from build123d import *

# Parameters (mm, degrees)
F0_W     = 50
F0_H     = 19
F0_H_2   = 13
F0_W_2   = 1.5
F1_DEPTH = 1.5
F2_R     = 0.74999
F4_DEPTH = 1.5
F5_R     = 1.49999
F3_W     = 2
F3_H     = 5
F6_DEPTH = 0.3


# Not quite as in the source:
# - a fillet or chamfer is up to 0.001 mm smaller than in the source, because OpenCascade refuses the exact size


with BuildPart() as f1:
    # F0 (on Top) → F1 (new body)
    with BuildSketch(Plane.XY):
        with Locations((0, -6.5)):
            Rectangle(F0_W, F0_H)
        with Locations((0, 9.5)):
            Rectangle(F0_W, F0_H_2)
        with Locations((-25.75, 9.5)):
            Rectangle(F0_W_2, F0_H_2)
        with Locations((25.75, 9.5)):
            Rectangle(F0_W_2, F0_H_2)
    extrude(amount=F1_DEPTH)

    # F2 (radius 0.75 in the source; OpenCascade refuses exactly that, so slightly less here)
    f2_edges = [f1.edges().sort_by_distance(p)[0] for p in [
        (-26.5, 16, 0.75),
        (-26.5, 3, 0.75),
        (-25, 3, 0.75),
        (-25, -16, 0.75),
        (25, -16, 0.75),
        (25, 3, 0.75),
        (26.5, 3, 0.75),
        (26.5, 16, 0.75),
    ]]
    fillet(f2_edges, radius=F2_R)

    # F3 (on face) → F4 (join)
    with BuildSketch(Plane.XY.offset(1.5)):
        Polygon((-23.5, 2.25), (-25, 2.25), (-25, -15.25), (-23.5, -15.25), (-23.5, -7), (-23.5, -2), align=None)
        Polygon((23.5, -15.25), (25, -15.25), (25, 2.25), (23.5, 2.25), (23.5, -2), (23.5, -7), align=None)
    extrude(amount=F4_DEPTH)

    # F5 (radius 1.5 in the source; OpenCascade refuses exactly that, so slightly less here)
    f5_edges = [f1.edges().sort_by_distance(p)[0] for p in [
        (-23.5, -6.5, 3),
        (23.5, -6.5, 3),
    ]]
    fillet(f5_edges, radius=F5_R)

    # F3 (on face) → F6 (join)
    with BuildSketch(Plane.XY.offset(1.5)):
        with Locations((-22.5, -4.5)):
            Rectangle(F3_W, F3_H)
        with Locations((22.5, -4.5)):
            Rectangle(F3_W, F3_H)
    extrude(amount=F6_DEPTH)


solid = f1.part
Work out the finished part from the listing and answer in its coordinate system (mm). A direction names the side the tool comes from. Give positions to 0.01 mm unless a question says otherwise; leave off trailing zeros. Order: outer loops, then holes, each group sorted by start corner. A loop starts at its lowest first (then second) coordinate and runs counter-clockwise, first axis right, second up. Notation, with made-up numbers: (-24.75, 43.5) -> (5.25, 43.5) arc R29 cw to (5.25, 68.5) -> close; hole circle Ø5 at (-6, -21). An arc over 180 degrees is marked (long way). Answer as a JSON object with one key per item and string values. Group by question number.
1. Section B-B on x = 22 is taken. Determine the outline of the cut face in (y, z), plus the area to 3 significant figures.
2. Section D-D on x = -7 is taken. Determine the outline of the cut face in (y, z), plus the area to 3 significant figures.
3. Flat-ended cylindrical pins translate along their axes: pin 1 Ø0.6 at (x, y) = (23, -4.5) entering from +Z; pin 2 Ø1.6 at (x, z) = (-24, 2.5) entering from +Y; pin 3 Ø16 at (x, y) = (4, -2) entering from +Z. Find the tip coordinate at first contact, or state that the pin passes through.
4. Consider line 1 along Z through (x, y) = (-17.5, -0.5); line 2 along X through (y, z) = (-4.5, 0.85); line 3 along X through (y, z) = (3.5, 0.1). Determine where each line is inside the solid, lowest interval first. Write a range as [from, to].
5. The mould has two halves that part along X. Classify faces 1 (the cylindrical face through (23.93, -6.62, 2.55)), 2 (the flat face through (-26.5, 9, 1)), 3 (the flat face through (0, 0, 0)), 4 (the flat face through (-23, -4, 1.8)): released by +X, released by -X, zero draft, split by the parting line, or undercut.
6. Section A-A on z = 2.5 is taken. Determine the outline of the cut face in (x, y).
7. A tool of negligible diameter and unlimited length cuts with its end or side. For faces 5 (the flat face through (24, 2.25, 2)), 6 (the flat face through (25, -7, 1)), 7 (the flat face through (-25, -6, 1)), from which of +Z, -Z, +X, -X, +Y, -Y can it reach the whole face along a straight path? Write none if from no direction.
Result sheet:
{
 "1": {"outline": "(-16, 0) -> (16, 0) -> (16, 1.5) -> (-2, 1.5) -> (-2, 1.8) -> (-7, 1.8) -> (-7, 1.5) -> (-16, 1.5) -> close", "area": "49.5 mm^2"},
 "2": {"outline": "(-16, 0) -> (16, 0) -> (16, 1.5) -> (-16, 1.5) -> close", "area": "48.0 mm^2"},
 "3": {"pin 1": "stops at z = 1.8", "pin 2": "stops at y = 2.25", "pin 3": "stops at z = 1.5"},
 "4": {"line 1": "z = [0, 1.5]", "line 2": "x = [-25, 25]", "line 3": "x = [-26.46, 26.46]"},
 "5": {"face 1": "undercut", "face 2": "released by -X", "face 3": "zero draft", "face 4": "undercut"},
 "6": {"outline": "(-25, -15.25) -> (-23.88, -15.25) -> (-23.88, 2.25) -> (-25, 2.25) -> close; (23.88, -15.25) -> (25, -15.25) -> (25, 2.25) -> (23.88, 2.25) -> close"},
 "7": {"face 5": "+Z, +X, -X, +Y", "face 6": "+Z, -Z, +X, -Y", "face 7": "+Z, -Z, -X, -Y"}
}
